Input: part model. Units: mm. Frame: model coordinates. A direction names the side the tool comes from. Coordinates: 2 decimals unless noted, no trailing zeros. Loops run counter-clockwise (first coordinate to the right, second up) from the corner with the lowest first, then second, coordinate; pieces in that order, holes last.
```python
from build123d import *

# Parameters (mm, degrees)
SKETCH_1_R           = 17
EXTRUDE_1_DEPTH      = 40
EXTRUDE_2_DEPTH      = 60
EXTRUDE_2_DEPTH_BACK = 20
SKETCH_2_W           = 41.02774957
SKETCH_2_H           = 100


with BuildPart() as part:
    # 草图1 → 凸台-拉伸1 (new body)
    with BuildSketch(Plane.XY):
        with BuildLine():
            ThreePointArc((-181.986125215, 315.209215145), (-315.209215145, 181.986125215), (-363.97225043, 0))
            Line((-363.97225043, 0), (-405, 0))
            ThreePointArc((-405, 0), (-350.740288533, 202.5), (-202.5, 350.740288533))
            ThreePointArc((-202.5, 350.740288533), (-174.477525913, 343.231689231), (-181.986125215, 315.209215145))
        make_face()
        with Locations((-192.243062607, 332.974751839)):
            Circle(SKETCH_1_R, mode=Mode.SUBTRACT)
    extrude(amount=EXTRUDE_1_DEPTH)

    # 草图2 → 凸台-拉伸2 (add, two sides: drawn at the far end of the back side and taken through both)
    with BuildSketch(Plane.XY.offset(-EXTRUDE_2_DEPTH_BACK)):
        with Locations((-384.486125215, -50)):
            Rectangle(SKETCH_2_W, SKETCH_2_H)
    extrude(amount=EXTRUDE_2_DEPTH + EXTRUDE_2_DEPTH_BACK)


solid = part.part
```
Item 1: Reachability of faces 1 (the face through (-363.972, -51, 19)), 2 (the face through (-385, 0, -10)), 3 (the face through (-322, 178, 40)), 4 (the face through (-385, -100, 19)), 5 (the face through (-352.215, 199.924, 19.72)) from +Z, -Z, +X, -X, +Y, -Y: full face, straight path, thin tool, end or side. Return the list, or none.
Result:
face 1: +Z, -Z, +X, -Y
face 2: -Z, +X, -X, +Y
face 3: +Z, +X, -X, +Y
face 4: +Z, -Z, +X, -X, -Y
face 5: +Z, -Z, -X, +Y
Item 2: Section query C-C (z = -9). Output: boundary loops of the cut face in (x, y).
Result:
outline: (-405, -100) - (-363.97, -100) - (-363.97, 0) - (-405, 0) - close
Item 3: Section query A-A (z = 18.5). Output: boundary loops of the cut face in (x, y).
Result:
outline: (-405, -100) - (-363.97, -100) - (-363.97, 0) arc R363.97 cw to (-181.99, 315.21) arc R20.51 ccw to (-202.5, 350.74) arc R405 ccw to (-405, 0) - close; hole circle Ø34 at (-192.24, 332.97)
Item 4: Contact query for flat-ended pins moving along their axis: P1, Ø6, axis at x = -352, y = 211.5, coming from the -Z side (3 decimals); P2, Ø3, axis at x = -223.5, z = 12.5, coming from the -Y side; P3, Ø5, axis at y = 289.5, z = 3, coming from the -X side; P4, Ø6, axis at x = -392, z = 52.5, coming from the +Y side. Output: stop coordinate, or through.
Result:
P1: passes through
P2: stops at y = 286.1
P3: stops at x = -285.76
P4: stops at y = 0
Item 5: Mould query, pull axis Y, two halves, no side actions, for faces 6 (the face through (-195.93, 316.38, 19.72)), 7 (the face through (-313.87, 184.29, 19.72)), 8 (the face through (-174.707, 343.62, 19.72)), 9 (the face through (-385, 0, 50)). Classes: +Y half, -Y half, draft (parallel to the pull), parting line (faces both ways), or undercut.
Result:
face 6: undercut
face 7: -Y half
face 8: parting line
face 9: +Y half
Item 6: Line query: L1, parallel to Y at x = -393, z = 48.5; L2, parallel to X at y = -15, z = 24; L3, parallel to Y at x = -206, z = 25.5. Output: solid intervals per line, ascending.
Result:
L1: y = -100 to 0
L2: x = -405 to -363.97
L3: y = 300.07 to 322.99, 342.96 to 348.7
Item 7: Section query B-B (y = -53). Output: boundary loops of the cut face in (x, z), then the cut area to 3 significant figures.
Result:
outline: (-405, -20) - (-363.97, -20) - (-363.97, 60) - (-405, 60) - close
area: 3,280 mm2
